Build history of the part. All positions in model axes, mm. Coordinates: 2 decimals unless noted, no trailing zeros. Loops run counter-clockwise (first coordinate to the right, second up) from the corner with the lowest first, then second, coordinate; pieces in that order, holes last.
(1) Wall check: L1, parallel to Z at x = 1068, y = 0; L2, parallel to X at y = -11, z = -67 (3 decimals); L3, parallel to Y at x = 1, z = -50. Give the ranges that are in metal, low to high.
(2) Flat gauge pins, fed straight in: P1, Ø20.5, axis at y = 0, z = -50.8, coming from the -X side; P2, Ø12, axis at x = 337.5, z = -10.5, coming from the -Y side; P3, Ø5, axis at x = 529, y = 10.5, coming from the -Z side; P4, Ø1.5, axis at x = 161.5, y = 7.5, coming from the -Z side. Where does each tip first touch, or does it go through?
(3) Slice it at C-C (x = 748). Give the cut face in (y, z) (3 decimals).
(4) Slice it at A-A (y = 0). Give the cut face in (x, z) (1 decimal).
(5) Slice it at B-B (z = 0). Give the cut face in (x, y) (3 decimals).
(6) Two-plate mould, pull along X, no slides. Class faces 1 (the face through (0, 0, 1)), 2 (the face through (3.175, 0, 18)), 3 (the face through (1069.975, 0, 1)): pulls with the +X half, pulls with the -X half, needs draft (parallel to the pull), parting line crosses it, or undercut.
from build123d import *

# Parameters (mm, degrees)
F0_R     = 15.875
F1_DEPTH = 1069.975
F2_W     = 38.1
F2_H     = 152.4
F3_DEPTH = 3.175
F5_D     = 15.875
F6_W     = 38.1
F6_H     = 152.4
F7_DEPTH = 3.175
F9_D     = 15.875


with BuildPart() as f1:
    # F0 (on Right) → F1 (new body)
    with BuildSketch(Plane.YZ):
        Circle(F0_R)
    extrude(amount=F1_DEPTH)

    # F2 (on Right) → F3 (join)
    with BuildSketch(Plane.YZ):
        Rectangle(F2_W, F2_H)
    extrude(amount=F3_DEPTH)

    # F5 (through all)
    with Locations(Plane.YZ.offset(1069.975)):
        with Locations((0, 50.8), (0, -50.8)):
            Hole(F5_D / 2)

    # F6 (on face) → F7 (join)
    with BuildSketch(Plane.YZ.offset(1069.975)):
        Rectangle(F6_W, F6_H)
    extrude(amount=-F7_DEPTH)

    # F9 (through all)
    with Locations(Plane(origin=(0, 0, 0), x_dir=(0, -1, 0), z_dir=(-1, 0, 0))):
        with Locations((0, 50.8), (0, -50.8)):
            Hole(F9_D / 2)


solid = f1.part
Response values:
1. L1: z = -76.2 to -58.74, -42.86 to 42.86, 58.74 to 76.2
1. L2: x = 0 to 3.175, 1066.8 to 1069.975
1. L3: y = -19.05 to -7.9, 7.9 to 19.05
2. P1: stops at x = 0
2. P2: stops at y = -15.22
2. P3: stops at z = -13.71
2. P4: stops at z = -14.37
3. outline: circle Ø31.75 at (0, 0)
4. outline: (0, -76.2) - (3.2, -76.2) - (3.2, -58.7) - (0, -58.7) - close; (0, -42.9) - (3.2, -42.9) - (3.2, -15.9) - (1066.8, -15.9) - (1066.8, -42.9) - (1070, -42.9) - (1070, 42.9) - (1066.8, 42.9) - (1066.8, 15.9) - (3.2, 15.9) - (3.2, 42.9) - (0, 42.9) - close; (0, 58.7) - (3.2, 58.7) - (3.2, 76.2) - (0, 76.2) - close; (1066.8, -76.2) - (1070, -76.2) - (1070, -58.7) - (1066.8, -58.7) - close; (1066.8, 58.7) - (1070, 58.7) - (1070, 76.2) - (1066.8, 76.2) - close
5. outline: (0, -19.05) - (3.175, -19.05) - (3.175, -15.875) - (1066.8, -15.875) - (1066.8, -19.05) - (1069.975, -19.05) - (1069.975, 19.05) - (1066.8, 19.05) - (1066.8, 15.875) - (3.175, 15.875) - (3.175, 19.05) - (0, 19.05) - close
6. face 1: pulls with the -X half
6. face 2: undercut
6. face 3: pulls with the +X half
